CAD build for the part. Positions are in the model's coordinates, mm. Give positions to 0.01 mm unless a question says otherwise; leave off trailing zeros. Order: outer loops, then holes, each group sorted by start corner. A loop starts at its lowest first (then second) coordinate and runs counter-clockwise, first axis right, second up. Notation, with made-up numbers: (-3, 89) -> (52, 89) arc R9 cw to (52, 98) -> close; hole circle Ø9 at (80, 66). An arc over 180 degrees is marked (long way). Answer as CSV lines item,"result".
```python
from build123d import *

# Parameters (mm, degrees)
F1_DEPTH = 15


with BuildPart() as f1:
    # F0 (on Top) → F1 (new body)
    with BuildSketch(Plane.XY):
        with BuildLine():
            ThreePointArc((23.5, 22.5), (13.5, 2.5), (3.5, 22.5))
            Line((3.5, 22.5), (2.275028, 22.5))
            ThreePointArc((2.275028, 22.5), (0.581271, 18.918729), (0, 15))
            Line((0, 15), (0, 0))
            Line((0, 0), (27, 0))
            Line((27, 0), (27, 15))
            ThreePointArc((27, 15), (26.418729, 18.918729), (24.724972, 22.5))
            Line((24.724972, 22.5), (23.5, 22.5))
        make_face()
    extrude(amount=F1_DEPTH)


solid = f1.part
```
1) Band-saw the part on A-A, the plane y = 20.5. Write the cut outline in (x, z), then the cut area to 3 significant figures.
Data:
outline,"(1.17, 0) -> (2.28, 0) -> (2.28, 15) -> (1.17, 15) -> close; (24.72, 0) -> (25.83, 0) -> (25.83, 15) -> (24.72, 15) -> close"
area,"33.1 mm2"
2) Band-saw the part on B-B, the plane z = 9.25. Write the cut outline in (x, y), then the cut area to 3 significant figures.
Data:
outline,"(0, 0) -> (27, 0) -> (27, 15) arc R13.5 ccw to (24.72, 22.5) -> (23.5, 22.5) arc R12.5 cw (long way) to (3.5, 22.5) -> (2.28, 22.5) arc R13.5 ccw to (0, 15) -> close"
area,"176 mm2"
3) Wall check: line 1 along X through (y, z) = (15, 7.75); line 2 along X through (y, z) = (16.5, 13.5); line 3 along Y through (x, z) = (2.75, 14). Give the ranges that are in metal, low to high. Write a range as [from, to].
Data:
line 1,"x = [0, 1], [26, 27]"
line 2,"x = [0.08, 1.09], [25.91, 26.92]"
line 3,"y = [0, 8.62], [21.38, 22.5]"
4) Band-saw the part on D-D, the plane x = 10.25. Write the cut outline in (y, z), then the cut area to 3 significant figures.
Data:
outline,"(0, 0) -> (2.93, 0) -> (2.93, 15) -> (0, 15) -> close"
area,"43.9 mm2"
5) Band-saw the part on C-C, the plane y = 4. Write the cut outline in (x, z), then the cut area to 3 significant figures.
Data:
outline,"(0, 0) -> (7.56, 0) -> (7.56, 15) -> (0, 15) -> close; (19.44, 0) -> (27, 0) -> (27, 15) -> (19.44, 15) -> close"
area,"227 mm2"
6) Pull direction X, two halves, no side cores. Call faces 1 (the cylindrical face through (13.887, 2.506, 7.395)), 2 (the cylindrical face through (26.435, 18.865, 7.395)), 3 (the flat face through (24, 22.5, 7)), 4 (the flat face through (0, 8, 7)): pulls with the +X half, pulls with the -X half, needs draft (parallel to the pull), parting line crosses it, or undercut.
Data:
face 1,"undercut"
face 2,"pulls with the +X half"
face 3,"needs draft"
face 4,"pulls with the -X half"
7) Pin check, flat tips, straight feed: P1, Ø2, axis at x = 4, y = 17, coming from the +Z side; P2, Ø4, axis at x = 9, z = 8, coming from the +Y side. Stop position of each tip, or through.
Data:
P1,"passes through"
P2,"stops at y = 4.32"
